Autodesk Inventor part; units mm, degrees
ref_plane "YZ Plane" through (0, 0, 0) normal (1, 0, 0) x (0, 1, 0)
ref_plane "XZ Plane" through (0, 0, 0) normal (0, 1, 0) x (-1, 0, 0)
ref_plane "XY Plane" through (0, 0, 0) normal (0, 0, 1) x (1, 0, 0)
sketch "スケッチ1" plane through (0, 0, 0) normal (0, 1, 0) x (-1, 0, 0)
  line L0 (12.5, 12.5) -> (-12.5, 12.5)
  line L1 (-12.5, 12.5) -> (-12.5, -12.5)
  line L2 (-12.5, -12.5) -> (12.5, -12.5)
  line L3 (12.5, -12.5) -> (12.5, 12.5)
  line L4 (10, -10) -> (-10, -10)
  line L5 (-10, -10) -> (-10, 10)
  line L6 (-10, 10) -> (10, 10)
  line L7 (10, 10) -> (10, -10)
  circle A0 centre (10, -10) radius 1.5
  circle A1 centre (-10, -10) radius 1.5
  circle A2 centre (-10, 10) radius 1.5
  circle A3 centre (10, 10) radius 1.5
  circle A4 centre (10, 10) radius 2.5
  circle A5 centre (-10, 10) radius 2.5
  circle A6 centre (-10, -10) radius 2.5
  circle A7 centre (10, -10) radius 2.5
  circle A8 centre (0, 0) radius 11.5
  circle A9 centre (0, 0) radius 7.5
  point P0 (12.5, 0)
  point P1 (0, -12.5)
  point P2 (-10, 0)
  point P3 (-12.5, 0)
  point P4 (0, -10)
  point P5 (12.5, 10)
  point P6 (10, 12.5)
  point P7 (-10, 12.5)
  point P8 (-12.5, 10)
  point P9 (-12.5, -10)
  point P10 (-10, -12.5)
  point P11 (10, -12.5)
  point P12 (12.5, -10)
  point P13 (-5.6789, 10)
  point P14 (5.6789, 10)
  dimension "d0" = 25
  dimension "d1" = 25
  dimension "d2" = 20
  dimension "d3" = 20
  dimension "d4" = 3
  dimension "d5" = 3
  dimension "d6" = 3
  dimension "d7" = 3
  dimension "d8" = 23
  dimension "d9" = 15
extrude "押し出し1" add sketch "スケッチ1" along normal blind 7 contours A4 L6 A8 A5 L0 | A4 L7 A3 L6 | L3 A7 L7 A8 A4 | A5 L6 A2 L5 | A4 L7 A8 L6 | L6 A3 L7 A4 | A7 L4 A0 L7 | A5 L5 A2 L6 | L6 A8 L5 A5 | A5 L5 A8 A6 L1 | A7 L4 A8 L7 | L7 A0 L4 A7 | L2 A6 L4 A8 A7 | A6 L5 A1 L4 | A6 L4 A1 L5 | L5 A8 L4 A6 | A9
sketch "スケッチ2" plane through (0, 7, 0) normal (0, 1, 0) x (1, 0, 0)
  circle A0 centre (0, 0) radius 7.5
  circle A1 centre (0, 0) radius 11.5
  line L0 (0, 7.5) -> (-2.1881, 11.2899)
  line L1 (0, 7.5) -> (4.3762, 7.5) construction
  line L2 (0, 11.5) -> (3.4783, 5.4754)
  line L3 (0, 11.5) -> (6.9566, 11.5) construction
  line L4 (-4.8209, 5.7453) -> (-8.9332, 7.2421)
  line L5 (-7.3921, 8.8095) -> (-0.855, 6.4302)
  line L6 (-7.3861, 1.3024) -> (-11.4984, -0.1944)
  line L7 (-11.3253, 1.997) -> (-4.7882, 4.3763)
  line L8 (-6.4952, -3.75) -> (-8.6833, -7.5399)
  line L9 (-9.9593, -5.75) -> (-6.481, 0.2746)
  line L10 (-2.5652, -7.0477) -> (-1.8052, -11.3574)
  line L11 (-3.9332, -10.8065) -> (-5.1412, -3.9555)
  line L12 (2.5652, -7.0477) -> (5.9175, -9.8607)
  line L13 (3.9332, -10.8065) -> (-1.3958, -6.3348)
  line L14 (6.4952, -3.75) -> (10.8714, -3.75)
  line L15 (9.9593, -5.75) -> (3.0027, -5.75)
  line L16 (7.3861, 1.3024) -> (10.7384, 4.1153)
  line L17 (11.3253, 1.997) -> (5.9962, -2.4747)
  line L18 (4.8209, 5.7453) -> (5.5808, 10.0551)
  line L19 (7.3921, 8.8095) -> (6.1841, 1.9586)
  point P0 (-2.5583, 7.0502)
  point P1 (-6.4916, 3.7563)
  point P2 (-7.3873, -1.2952)
  point P3 (-4.8265, -5.7407)
  point P4 (-0.0073, -7.5)
  point P5 (4.8153, -5.75)
  point P6 (7.3848, -1.3095)
  point P7 (6.4988, 3.7437)
  point P8 (2.572, 7.0452)
  dimension "d12" = 120
  dimension "d13" = 60
  dimension "d16" = 360
extrude "押し出し2" add sketch "スケッチ2" against normal up to surface (7 mm away) contours A0 L16 A1 L17 | A0 L18 A1 L19 | L14 A1 L15 A0 | A0 L0 A1 L2 | L12 A1 L13 A0 | A0 L4 A1 L5 | L10 A1 L11 A0 | A0 L6 A1 L7 | L8 A1 L9 A0
properties part number "Fan"
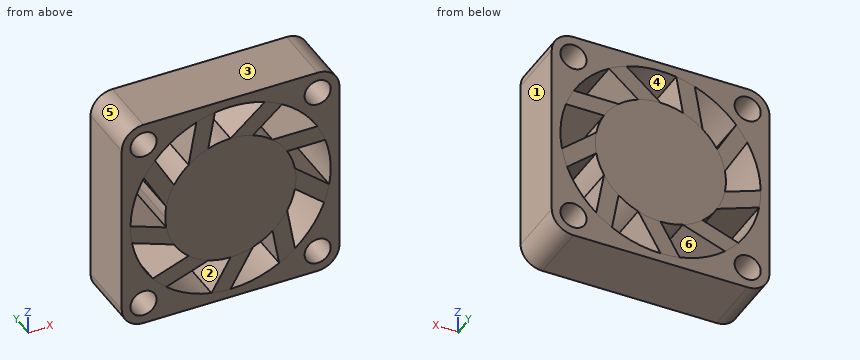
Check sheet for the modelled part. Datum: model origin and axes. Units: mm. Face numbers are marked on the shaded views. A direction names the side the tool comes from. Round coordinates to 2 decimals unless told otherwise and drop trailing zeros. Loops run counter-clockwise (first coordinate to the right, second up) from the corner with the lowest first, then second, coordinate; pieces in that order, holes last. Notation, with made-up numbers: M 27.25,32 L 84.25,32 A19 ccw 84.25,56 Z; hole C 57,2 d9. An arc over 180 degrees is marked long. Answer as a JSON object with one key per item and string values.
1. Section check B-B (z = 3.25). Record the boundary of the cut face in (x, y).
Reply:
{"outline": "M -12.5,0 L -11.03,0 L -11.03,7 L -12.5,7 Z; M -8.52,0 L 6.76,0 L 6.76,7 L -8.52,7 Z; M 11.03,0 L 12.5,0 L 12.5,7 L 11.03,7 Z"}
2. Section check D-D (y = 2.5). State how many separate pieces and enclosed holes the cut face has, plus the area to 3 significant figures.
Reply:
{"separate pieces": "1", "enclosed holes": "13", "area": "437 mm²"}
3. Access from +Z, -Z, +X, -X, +Y, -Y to the whole of each face (thin tool, end or side, straight path). Record for the marked faces 5 and 6.
Reply:
{"face 5": "+Z, -X, +Y, -Y", "face 6": "+Y, -Y"}
4. Section check A-A (z = -10.5). Record the boundary of the cut face in (x, y).
Reply:
{"outline": "M -12.45,0 L -11.41,0 L -11.41,7 L -12.45,7 Z; M -8.59,0 L -4.69,0 L -4.69,7 L -8.59,7 Z; M -1.73,0 L 0.58,0 L 0.58,7 L -1.73,7 Z; M 4.69,0 L 8.59,0 L 8.59,7 L 4.69,7 Z; M 11.41,0 L 12.45,0 L 12.45,7 L 11.41,7 Z"}
5. Section check C-C (x = 5.25). Record the boundary of the cut face in (y, z).
Reply:
{"outline": "M 0,-12.5 L 7,-12.5 L 7,-10.23 L 0,-10.23 Z; M 0,-8.18 L 7,-8.18 L 7,5.75 L 0,5.75 Z; M 0,9.3 L 7,9.3 L 7,12.5 L 0,12.5 Z"}
6. Gauge pin test, flat end, axial feed: P1, Ø1.8, axis at x = -10, z = -10, coming from the -Y side. Record the tip position at first contact, or that the pin passes through.
Reply:
{"P1": "passes through"}
7. Scan lines: line 1 (X direction, y = 2.75, z = 4.5); line 2 (Z direction, x = -5.25, y = 2); line 3 (Z direction, x = -10, y = 2.75). Record each from-to range of solid material in increasing order.
Reply:
{"line 1": "x = -12.5 to -10.58, -9.24 to -6.93, -6 to 12.5", "line 2": "z = -12.5 to -10.23, -8.03 to -5.9, -5.36 to 5.36, 10.23 to 12.5", "line 3": "z = -12.5 to -11.5, -8.5 to -5.68, -2.48 to -0.35, 5.68 to 8.5, 11.5 to 12.5"}
8. Mould release check, pull along X, two halves, no side actions. Record for the marked faces 1, 2, 3 and 4: pulls with the +X half, pulls with the -X half, needs draft (parallel to the pull), parting line crosses it, or undercut.
Reply:
{"face 1": "pulls with the +X half", "face 2": "undercut", "face 3": "needs draft", "face 4": "undercut"}
